Read the model definition and answer for the solid it produces. Units are mm, in the model's axes. Coordinates: 2 decimals unless noted, no trailing zeros. Write each loop counter-clockwise with the first axis right and the second up, starting at its lowest first coordinate (ties: lowest second). Pieces come first, ordered by that corner, then holes. Notation, with made-up numbers: (51.5, 25.5) -> (104.5, 25.5) arc R29 cw to (104.5, 57.5) -> close; hole circle Ø3 at (0, 83). An arc over 180 degrees is marked (long way). One line per item, written item: value. Start each with the question number.
1. Find section B-B, the plane y = 9. Write down the section's boundary in (x, z), and give its area (3 significant figures).
2. Consider line 1 along Y through (x, z) = (-70, 0.7); line 2 along X through (y, z) = (9, 4.1); line 3 along Y through (x, z) = (-19.5, 2.8). Determine where each line is inside the solid, lowest interval first.
3. Find section A-A, the plane x = -76.5. Write down the section's boundary in (y, z).
4. Given P1, Ø1, axis at x = -56, y = 52.5, coming from the -Z side; P2, Ø4, axis at x = 32.96, y = 49.34, coming from the -Z side, each flat-ended and moving along its own axis, determine where each tip first touches the part or whether it passes through.
5. Find section C-C, the plane z = 3.55. Write down the section's boundary in (x, y) (3 decimals), and give its area (3 significant figures).
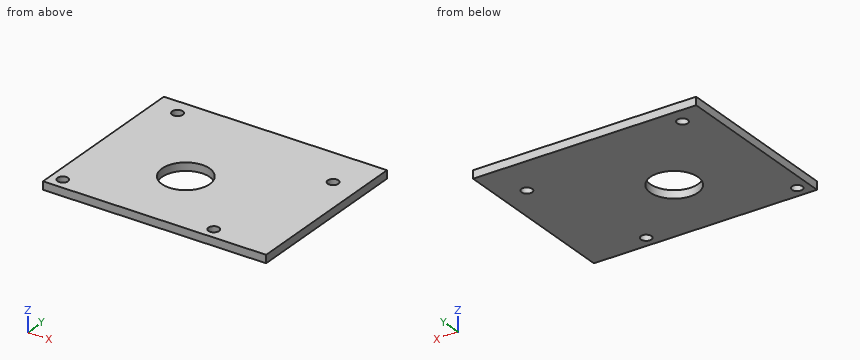
```python
from build123d import *

# Parameters (mm, degrees)
SKETCH1_W           = 133
SKETCH1_H           = 105
SKETCH1_R           = 14.225
BOSS_EXTRUDE2_DEPTH = 4.7625
CUT_EXTRUDE1_REACH  = 115.05
SKETCH2_R           = 3.18


with BuildPart() as part:
    # Sketch1 → Boss-Extrude2 (new body)
    with BuildSketch(Plane.XY):
        with Locations((-18.535460993, 21.841271178)):
            Rectangle(SKETCH1_W, SKETCH1_H)
        with Locations(Location((-30.035460993, 13.261258957, 0), (0, 0, 180))):
            Circle(SKETCH1_R, mode=Mode.SUBTRACT)
    extrude(amount=BOSS_EXTRUDE2_DEPTH)

    # Sketch2 → Cut-Extrude1 (cut, up to next)
    with BuildSketch(Plane.XY.offset(4.7625), mode=Mode.PRIVATE) as cut_extrude1_sk1:
        with Locations((-70.035460993, 64.341271178)):
            Circle(SKETCH2_R)
    cut_extrude1_tool1 = extrude(cut_extrude1_sk1.sketch, amount=-CUT_EXTRUDE1_REACH, mode=Mode.PRIVATE) & part.part
    # Sketch2 → Cut-Extrude1 (cut, up to next)
    with BuildSketch(Plane.XY.offset(4.7625), mode=Mode.PRIVATE) as cut_extrude1_sk2:
        with Locations((32.964539007, 49.341271178)):
            Circle(SKETCH2_R)
    cut_extrude1_tool2 = extrude(cut_extrude1_sk2.sketch, amount=-CUT_EXTRUDE1_REACH, mode=Mode.PRIVATE) & part.part
    # Sketch2 → Cut-Extrude1 (cut, up to next)
    with BuildSketch(Plane.XY.offset(4.7625), mode=Mode.PRIVATE) as cut_extrude1_sk3:
        with Locations((11.964539007, -23.658728822)):
            Circle(SKETCH2_R)
    cut_extrude1_tool3 = extrude(cut_extrude1_sk3.sketch, amount=-CUT_EXTRUDE1_REACH, mode=Mode.PRIVATE) & part.part
    # Sketch2 → Cut-Extrude1 (cut, up to next)
    with BuildSketch(Plane.XY.offset(4.7625), mode=Mode.PRIVATE) as cut_extrude1_sk4:
        with Locations((-78.035460993, -23.658728822)):
            Circle(SKETCH2_R)
    cut_extrude1_tool4 = extrude(cut_extrude1_sk4.sketch, amount=-CUT_EXTRUDE1_REACH, mode=Mode.PRIVATE) & part.part
    add(cut_extrude1_tool1.solids().sort_by_distance((-70.035461, 64.341271, 4.7625))[0], mode=Mode.SUBTRACT)
    add(cut_extrude1_tool2.solids().sort_by_distance((32.964539, 49.341271, 4.7625))[0], mode=Mode.SUBTRACT)
    add(cut_extrude1_tool3.solids().sort_by_distance((11.964539, -23.658729, 4.7625))[0], mode=Mode.SUBTRACT)
    add(cut_extrude1_tool4.solids().sort_by_distance((-78.035461, -23.658729, 4.7625))[0], mode=Mode.SUBTRACT)


solid = part.part
```
Answer block:
1. outline: (-85.04, 0) -> (-43.61, 0) -> (-43.61, 4.76) -> (-85.04, 4.76) -> close; (-16.46, 0) -> (47.96, 0) -> (47.96, 4.76) -> (-16.46, 4.76) -> close
1. area: 504 mm2
2. line 1: y = -30.66 to 61.16, 67.52 to 74.34
2. line 2: x = -85.04 to -43.61, -16.46 to 47.96
2. line 3: y = -30.66 to 3.7, 22.82 to 74.34
3. outline: (-30.66, 0) -> (-26.44, 0) -> (-26.44, 4.76) -> (-30.66, 4.76) -> close; (-20.87, 0) -> (74.34, 0) -> (74.34, 4.76) -> (-20.87, 4.76) -> close
4. P1: stops at z = 0
4. P2: passes through
5. outline: (-85.035, -30.659) -> (47.965, -30.659) -> (47.965, 74.341) -> (-85.035, 74.341) -> close; hole circle Ø6.36 at (-78.035, -23.659); hole circle Ø6.36 at (-70.035, 64.341); hole circle Ø28.45 at (-30.035, 13.261); hole circle Ø6.36 at (11.965, -23.659); hole circle Ø6.36 at (32.965, 49.341)
5. area: 13,200 mm2
